Check sheet for the modelled part. Datum: model origin and axes. Units: mm. Face numbers are marked on the shaded views. A direction names the side the tool comes from. Round coordinates to 2 decimals unless told otherwise and drop trailing zeros. Loops run counter-clockwise (first coordinate to the right, second up) from the corner with the lowest first, then second, coordinate; pieces in that order, holes last. Notation, with made-up numbers: (21, 71) -> (25, 71) arc R17 ccw to (25, 100) -> close; hole circle Ø6 at (71.25, 89). An arc over 180 degrees is marked (long way). Return JSON: item names as keys, results as strings.
from build123d import *

# Parameters (mm, degrees)
BOSS_EXTRUDE1_DEPTH = 2.5
SKETCH6_R           = 1.75
SKETCH6_W           = 10.8
SKETCH6_H           = 10.8
CUT_EXTRUDE1_DEPTH  = 50.137003564
FILLET1_R           = 5.4
FILLET2_R           = 5.4
FILLET3_RADIUS      = 10
FILLET3_LENGTH      = 2.5
SKETCH7_W           = 35
SKETCH7_H           = 20
SKETCH7_W_2         = 23
SKETCH7_H_2         = 13
BOSS_EXTRUDE2_DEPTH = 6.5
CUT_EXTRUDE2_DEPTH  = 5.5
FILLET4_R           = 4
SKETCH9_W           = 2.5
SKETCH9_H           = 24
BOSS_EXTRUDE3_DEPTH = 35
SKETCH11_R          = 3.5
SKETCH11_R_2        = 0.5
CUT_EXTRUDE3_DEPTH  = 72.106548013
FILLET5_R           = 5
BOSS_EXTRUDE4_DEPTH = 2.5
CUT_EXTRUDE5_DEPTH  = 73.478504536
SKETCH17_W          = 5.3
SKETCH17_H          = 13
SKETCH17_R          = 0.75
BOSS_EXTRUDE5_DEPTH = 6.5
BOSS_EXTRUDE6_DEPTH = 9
SKETCH22_W          = 12.144268415
SKETCH22_H          = 32.489830624
CUT_EXTRUDE11_DEPTH = 75.735546033
FILLET11_R          = 5
SKETCH23_R          = 0.75
CUT_EXTRUDE12_DEPTH = 6.5
FILLET12_R          = 4
SKETCH24_W          = 4.9
SKETCH24_H          = 13
CUT_EXTRUDE13_DEPTH = 6.5
SKETCH26_W          = 22.6
SKETCH26_H          = 13
CUT_EXTRUDE14_DEPTH = 10
SKETCH29_W          = 6
SKETCH29_H          = 20
CUT_EXTRUDE15_DEPTH = 6.5
FILLET13_R          = 2
FILLET14_R          = 2


# Some blends are built 0.0001 mm under size
with BuildPart() as part:
    # Sketch1 → Boss-Extrude1 (new body)
    with BuildSketch(Plane.XY):
        Polygon((17.783093717, 10), (17.783093717, -10), (-6.22432909, -10), (-16.225555947, -25.001878594), (-32.225555947, -25.001878594), (-42.226782805, -10), (-42.221702947, 4.99999914), (-32.215396169, 19.998489886), (-16.215396169, 19.998489886), (-6.216906283, 10), align=None)
    extrude(amount=BOSS_EXTRUDE1_DEPTH)

    # Sketch6 → Cut-Extrude1 (cut, through all)
    with BuildSketch(Plane.XY.offset(2.5)):
        with Locations((-37.223395946, 0)):
            Circle(SKETCH6_R)
        with Locations((-32.225555947, -20.001878594)):
            Circle(SKETCH6_R)
        with Locations((-16.225555947, -20.001878594)):
            Circle(SKETCH6_R)
        with Locations((-10.316906283, 0)):
            Rectangle(SKETCH6_W, SKETCH6_H)
    extrude(amount=-CUT_EXTRUDE1_DEPTH, mode=Mode.SUBTRACT)

    # Fillet1
    fillet1_edges = [part.edges().sort_by_distance(p)[0] for p in [
        (-15.716906283, -5.4, 1.25),
        (-15.716906283, 5.4, 1.25),
    ]]
    fillet(fillet1_edges, radius=FILLET1_R - 0.0001)  # a hair under: the kernel refuses the full size

    # Fillet2
    # the kernel refuses this fillet: 5.4 mm, written as the material it adds along each edge
    with BuildSketch(Plane(origin=(-4.916906283, 5.4, 2.5), x_dir=(0, -1, 0), z_dir=(0, 0, -1)), Plane(origin=(-4.916906283, -5.4, 2.5), x_dir=(-1, 0, 0), z_dir=(0, 0, -1))) as fillet2_piece_1:
        with BuildLine():
            CenterArc((FILLET2_R, FILLET2_R), FILLET2_R, 180, 90)
            Line((0, FILLET2_R), (0, 0))
            Line((0, 0), (FILLET2_R, 0))
        make_face()
    extrude(amount=2.5)
    # the kernel refuses this fillet: 5.4 mm, written as the material it takes off along each edge

    # Fillet3: full round fillet: the end face becomes a half cylinder, R = half its width
    fillet3_face = Plane((17.783093717, 0, 1.25), x_dir=(0, 0, 1), z_dir=(1, 0, 0))  # on the end face: x along it, z out of the body
    fillet3_slab = fillet3_face.offset(-FILLET3_RADIUS / 2) * Box(FILLET3_LENGTH, 2 * FILLET3_RADIUS, FILLET3_RADIUS, mode=Mode.PRIVATE)  # the body's end, R deep
    fillet3_round = Plane((7.783093717, 0, 1.25), x_dir=(1, 0, 0), z_dir=(0, 0, 1)) * Cylinder(FILLET3_RADIUS, FILLET3_LENGTH, mode=Mode.PRIVATE)  # its axis R under the face
    add(fillet3_slab - fillet3_round, mode=Mode.SUBTRACT)

    # Sketch7 → Boss-Extrude2 (add)
    with BuildSketch(Plane.XY.offset(2.5)):
        with Locations((-10.316906283, 0)):
            Rectangle(SKETCH7_W, SKETCH7_H)
        with Locations((-10.316906283, 0)):
            Rectangle(SKETCH7_W_2, SKETCH7_H_2, mode=Mode.SUBTRACT)
    extrude(amount=BOSS_EXTRUDE2_DEPTH)

    # Sketch8 → Cut-Extrude2 (cut)
    with BuildSketch(Plane.XY.offset(2.5)):
        with BuildLine():
            Line((7.183093717, 10), (7.183093717, -10))
            Line((7.183093717, -10), (7.783093717, -10))
            ThreePointArc((7.783093717, -10), (17.783093717, 0), (7.783093717, 10))
            Line((7.783093717, 10), (7.183093717, 10))
        make_face()
    extrude(amount=-CUT_EXTRUDE2_DEPTH, mode=Mode.SUBTRACT)

    # Fillet4
    fillet4_edges = [part.edges().sort_by_distance(p)[0] for p in [
        (7.183093717, -10, 4.5),
        (7.183093717, 10, 4.5),
    ]]
    fillet(fillet4_edges, radius=FILLET4_R)

    # Sketch9 → Boss-Extrude3 (add)
    with BuildSketch(Plane(origin=(0, 19.998489886, 0), x_dir=(1, 0, 0), z_dir=(0, 1, 0))):
        with Locations((-32.215396169, -12)):
            Rectangle(SKETCH9_W, SKETCH9_H)
    extrude(amount=BOSS_EXTRUDE3_DEPTH)

    # Sketch11 → Cut-Extrude3 (cut, through all)
    with BuildSketch(Plane(origin=(-30.965396169, 0, 0), x_dir=(0, 0, -1), z_dir=(1, 0, 0))):
        with Locations(Location((-10, 40.998489886, 0), (0, 0, 90))):
            Circle(SKETCH11_R)
        with Locations(Location((-10, 32.998489886, 0), (0, 0, 90))):
            Circle(SKETCH11_R_2)
    extrude(amount=-CUT_EXTRUDE3_DEPTH, mode=Mode.SUBTRACT)

    # Fillet5
    fillet5_edges = [part.edges().sort_by_distance(p)[0] for p in [
        (-32.215396169, 54.998489886, 0),
        (-32.215396169, 54.998489886, 24),
    ]]
    fillet(fillet5_edges, radius=FILLET5_R)

    # Sketch14 → Boss-Extrude4 (add)
    with BuildSketch(Plane(origin=(-30.965396169, 0, 0), x_dir=(0, 0, -1), z_dir=(1, 0, 0))):
        Polygon((-24, 19.998489886), (-10.54641456, 9.845474641), (0, 9.845474641), (0, 19.998489886), align=None)
    extrude(amount=-BOSS_EXTRUDE4_DEPTH)

    # Sketch16 → Cut-Extrude5 (cut, through all)
    with BuildSketch(Plane.ZY.offset(33.465396169)):
        Polygon((10.54641456, 9.845474641), (24, 29.998489886), (24, 19.998489886), align=None)
    extrude(amount=-CUT_EXTRUDE5_DEPTH, mode=Mode.SUBTRACT)

    # Sketch17 → Boss-Extrude5 (add)
    with BuildSketch(Plane.XY.offset(2.5)):
        with Locations((-19.166906283, 0)):
            Rectangle(SKETCH17_W, SKETCH17_H)
        with Locations(Location((-19.166906283, 0, 0), (0, 0, 180))):
            Circle(SKETCH17_R, mode=Mode.SUBTRACT)
    extrude(amount=BOSS_EXTRUDE5_DEPTH)

    # Sketch18 → Boss-Extrude6 (add)
    with BuildSketch(Plane.XY.offset(9)):
        with BuildLine():
            Line((3.183093717, 10), (11.083093717, 10))
            Line((11.083093717, 10), (11.083093717, -10))
            Line((11.083093717, -10), (3.183093717, -10))
            ThreePointArc((3.183093717, -10), (6.011520842, -8.828427125), (7.183093717, -6))
            Line((7.183093717, -6), (7.183093717, 6))
            ThreePointArc((7.183093717, 6), (6.011520842, 8.828427125), (3.183093717, 10))
        make_face()
    extrude(amount=-BOSS_EXTRUDE6_DEPTH)

    # Sketch22 → Cut-Extrude11 (cut, through all)
    with BuildSketch(Plane.ZY.offset(33.465396169)):
        with Locations((25.072134207, 38.753574574)):
            Rectangle(SKETCH22_W, SKETCH22_H)
    extrude(amount=-CUT_EXTRUDE11_DEPTH, mode=Mode.SUBTRACT)

    # Fillet11
    fillet11_edges = [part.edges().sort_by_distance(p)[0] for p in [
        (-32.215396169, 54.998489886, 19),
        (-32.215396169, 22.508659262, 19),
    ]]
    fillet(fillet11_edges, radius=FILLET11_R)

    # Sketch23 → Cut-Extrude12 (cut)
    with BuildSketch(Plane.XY.offset(9)):
        with Locations((8.433093717, 0)):
            Circle(SKETCH23_R)
    extrude(amount=-CUT_EXTRUDE12_DEPTH, mode=Mode.SUBTRACT)

    # Fillet12
    fillet12_edges = [part.edges().sort_by_distance(p)[0] for p in [
        (11.083093717, -10, 4.5),
        (11.083093717, 10, 4.5),
    ]]
    fillet(fillet12_edges, radius=FILLET12_R)

    # Sketch24 → Cut-Extrude13 (cut)
    with BuildSketch(Plane.XY.offset(9)):
        with Locations((3.633093717, 0)):
            Rectangle(SKETCH24_W, SKETCH24_H)
    extrude(amount=-CUT_EXTRUDE13_DEPTH, mode=Mode.SUBTRACT)

    # Sketch26 → Cut-Extrude14 (cut)
    with BuildSketch(Plane.XY.offset(2.5)):
        with Locations((-5.216906283, 0)):
            Rectangle(SKETCH26_W, SKETCH26_H)
    extrude(amount=-CUT_EXTRUDE14_DEPTH, mode=Mode.SUBTRACT)

    # Sketch29 → Cut-Extrude15 (cut)
    with BuildSketch(Plane.XY.offset(9)):
        with Locations((-24.816906283, 0)):
            Rectangle(SKETCH29_W, SKETCH29_H)
    extrude(amount=-CUT_EXTRUDE15_DEPTH, mode=Mode.SUBTRACT)

    # Fillet13
    fillet13_edges = [part.edges().sort_by_distance(p)[0] for p in [
        (-6.22432909, -10, 1.25),
        (-16.225555947, -25.001878594, 1.25),
        (-32.225555947, -25.001878594, 1.25),
        (-42.226782805, -10, 1.25),
        (-42.221702947, 4.99999914, 1.25),
        (-16.215396169, 19.998489886, 1.25),
        (-6.216906283, 10, 1.25),
        (-33.465396169, 18.124860199, 1.25),
        (-14.020617686, -10, 2.5),
        (-21.816906283, -10, 5.75),
        (-21.816906283, 0, 2.5),
        (-21.816906283, 10, 5.75),
        (-14.016906283, 10, 2.5),
    ]]
    fillet(fillet13_edges, radius=FILLET13_R)

    # Fillet14
    fillet14_edges = [part.edges().sort_by_distance(p)[0] for p in [
        (-32.215396169, 9.845474641, 10.54641456),
    ]]
    fillet(fillet14_edges, radius=FILLET14_R)


solid = part.part
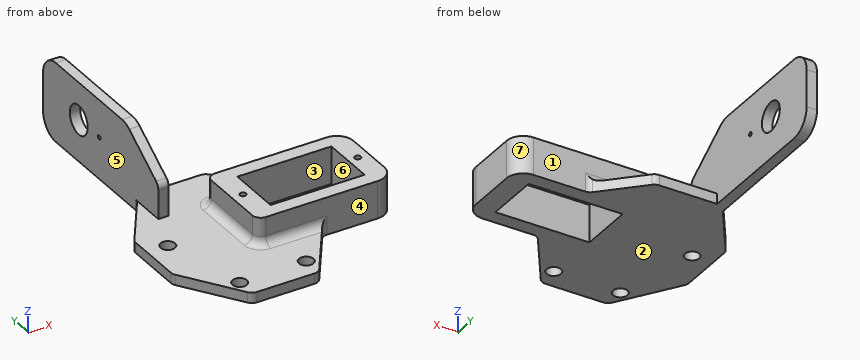
Q1. Material ranges on line 1 (Y direction, x = 5, z = 7.25); line 2 (X direction, y = 47.5, z = 6.25); line 3 (X direction, y = 3.5, z = 5.5), recorded low to high.
Results list:
{"line 1": "-10 to -6.5, 6.5 to 10", "line 2": "-33.47 to -30.97", "line 3": "-21.82 to -16.52, 6.08 to 11.08"}
Q2. Tool access check on the marked faces 1, 2, 3 and 4. Record the directions out of +Z, -Z, +X, -X, +Y, -Y that give a thin tool (end or side, any length) a straight path to the whole face; none if there is none.
Results list:
{"face 1": "+Z, +X, +Y", "face 2": "-Z, +X, -X, +Y, -Y", "face 3": "+Z, -Z", "face 4": "+Z, +X, -Y"}
Q3. Section check C-C (y = 29). Record the boundary of the cut face in (x, z).
Results list:
{"outline": "(-33.47, 0) -> (-30.97, 0) -> (-30.97, 19) -> (-33.47, 19) -> close"}
Q4. Section check D-D (z = 15.5). Record the boundary of the cut face in (x, y).
Results list:
{"outline": "(-33.47, 17.27) -> (-30.97, 17.27) -> (-30.97, 54.77) -> (-33.47, 54.77) -> close"}
Q5. Go/stop test with flat-tipped pins: pin 1 (3 mm diameter, centred on y = 39, z = 5, fed in from +X); pin 2 (3 mm diameter, centred on y = -3, z = 6, fed in from -X); pin 3 (4.5 mm diameter, centred on x = -32.23, y = -20, fed in from +Z); pin 4 (4 mm diameter, centred on x = -25.5, y = -12, fed in from -Z). Record where each tip stops, or that it passes through.
Results list:
{"pin 1": "x = -30.97", "pin 2": "x = -21.82", "pin 3": "z = 2.5", "pin 4": "z = 0"}
Q6. Section check A-A (x = 2.5). Record the boundary of the cut face in (y, z).
Results list:
{"outline": "(-10, 0) -> (-6.5, 0) -> (-6.5, 9) -> (-10, 9) -> close; (6.5, 0) -> (10, 0) -> (10, 9) -> (6.5, 9) -> close"}
Q7. Section check B-B (x = -12). Record the boundary of the cut face in (y, z).
Results list:
{"outline": "(-18.66, 0) -> (-6.5, 0) -> (-6.5, 9) -> (-10, 9) -> (-10, 4.5) arc R2 cw to (-12, 2.5) -> (-18.66, 2.5) -> close; (6.5, 0) -> (15.78, 0) -> (15.78, 2.5) -> (12, 2.5) arc R2 cw to (10, 4.5) -> (10, 9) -> (6.5, 9) -> close"}
Q8. Draft check along Y on the marked faces 5, 6 and 7. Enter one of: released by +Y, released by -Y, zero draft, split by the parting line, or undercut.
Results list:
{"face 5": "zero draft", "face 6": "undercut", "face 7": "released by +Y"}
